```python
from build123d import *

# Parameters (mm, degrees)
SKETCH006_W   = 11.8
SKETCH006_H   = 11.8
PAD006_DEPTH  = 30
SKETCH001_R   = 40
SKETCH001_R_2 = 2.1
PAD001_DEPTH  = 5
PAD004_DEPTH  = 10.5
SKETCH005_R   = 2.1
PAD005_DEPTH  = 20
SKETCH_W      = 11.8
SKETCH_H      = 11.8
PAD_DEPTH     = 15


with BuildPart() as pad006:
    # Sketch006 → Pad006 (new body)
    with BuildSketch(Plane.XY):
        Rectangle(SKETCH006_W, SKETCH006_H)
    extrude(amount=PAD006_DEPTH)


with BuildPart() as pad001:
    # Sketch001 → Pad001 (new body)
    with BuildSketch(Plane.XY):
        Circle(SKETCH001_R)
        with Locations((0, 35)):
            Circle(SKETCH001_R_2, mode=Mode.SUBTRACT)
        with Locations((-35, 0)):
            Circle(SKETCH001_R_2, mode=Mode.SUBTRACT)
        with Locations((35, 0)):
            Circle(SKETCH001_R_2, mode=Mode.SUBTRACT)
        with Locations((0, -35)):
            Circle(SKETCH001_R_2, mode=Mode.SUBTRACT)
    extrude(amount=PAD001_DEPTH)


with BuildPart() as vis:
    # Cone → Cone (revolve)
    with BuildSketch(Plane(origin=(0, 0, 5), x_dir=(1, 0, 0), z_dir=(0, -1, 0))):
        Polygon((0, 0), (30, 0), (11.9, 9), (0, 9), align=None)
    revolve(axis=Axis((0, 0, 5), (0, 0, 1)))

    # Fusion001: union Pad001
    add(pad001.part)

    # Cut001: cut Pad006
    add(pad006.part, mode=Mode.SUBTRACT)


with BuildPart() as pad004:
    # Sketch004 → Pad004 (new body)
    with BuildSketch(Plane.XZ):
        Polygon((4.25, 24), (2.125, 27.680608), (-2.125, 27.680608), (-4.25, 24), (-2.125, 20.319392), (2.125, 20.319392), align=None)
    extrude(amount=PAD004_DEPTH)


with BuildPart() as screw_hole:
    # Sketch005 → Pad005 (new body)
    with BuildSketch(Plane.XZ):
        with Locations((0, 24)):
            Circle(SKETCH005_R)
    extrude(amount=PAD005_DEPTH)

    # Fusion: union Pad004
    add(pad004.part)


with BuildPart() as mobile:
    # Sketch → Pad (new body)
    with BuildSketch(Plane.XY.offset(15)):
        with BuildLine():
            ThreePointArc((7.5, -9.239048), (0, 11.9), (-7.5, -9.239048))
            Line((-7.5, -9.239048), (-7.5, -13.239048))
            Line((-7.5, -13.239048), (7.5, -13.239048))
            Line((7.5, -13.239048), (7.5, -9.239048))
        make_face()
        Rectangle(SKETCH_W, SKETCH_H, mode=Mode.SUBTRACT)
    extrude(amount=PAD_DEPTH)

    # Cut: cut screw_hole
    add(screw_hole.part, mode=Mode.SUBTRACT)


with BuildPart() as mobile_1:
    # Cut placement: moved
    add(mobile.part.moved(Location((0, 0, -4))))

    # Fusion002: union vis
    add(vis.part)


solid = mobile_1.part
```
The listing builds one solid part. Answer for the finished solid, in the listing's coordinates (mm). A direction names the side the tool comes from. Give positions to 0.01 mm unless a question says otherwise; leave off trailing zeros. Loops run counter-clockwise (first coordinate to the right, second up) from the corner with the lowest first, then second, coordinate; pieces in that order, holes last. Notation, with made-up numbers: (-36.5, 2) - (-6.5, 2) arc R24 cw to (-6.5, 17) - close; hole circle Ø4 at (64.5, 61). An arc over 180 degrees is marked (long way). Answer as CSV lines item,"result". Start each with the question number.
Item 1: A cutting plane is placed at D-D on y = -35. Determine the outline of the cut face in (x, z), then the cut area to 3 significant figures.
Item 2: A cutting plane is placed at C-C on x = 0. Count the separate pieces of the cut face and the enclosed holes in it, then the cut area to 3 significant figures.
Item 3: A cutting plane is placed at A-A on z = 24.75. Determine the outline of the cut face in (x, y), then the cut area to 3 significant figures.
Item 4: For faces 1 (the face through (0, 5.9, 13)), 2 (the face through (3.202, -8.168, 21.815)), 3 (the face through (0.41, 11.893, 19.916)), 4 (the face through (1.13, -11.85, 21.77)), determine the directions among +Z, -Z, +X, -X, +Y, -Y from which every point of the face is accessible in a straight line to the end or side of a thin tool.
Item 5: A cutting plane is placed at B-B on y = 0. Determine the outline of the cut face in (x, z), then the cut area to 3 significant figures.
Item 6: Each of these flat-tipped pins is pushed along its axis until it touches: pin 1 (1 mm diameter, centred on x = -1, y = 14.5, fed in from +Z); pin 2 (3.5 mm diameter, centred on x = 2, z = 19.5, fed in from +Y); pin 3 (13 mm diameter, centred on x = 2.5, z = 7, fed in from -Y); pin 4 (3.5 mm diameter, centred on x = 0, y = -35, fed in from -Z). Where does it stop, or does it pass through?
Item 7: The mould has two halves that part along Z. Classify faces 5 (the face through (9, -29, 5)), 6 (the face through (-7.5, -11, 19)), 7 (the face through (0, -8, 16.319)): +Z half, -Z half, draft (parallel to the pull), parting line (faces both ways), or undercut.
Item 8: Find the intervals of material crossed by line 1 (Y direction, x = 0, z = 2.8); line 2 (Z direction, x = 0, y = -11); line 3 (X direction, y = -0.5, z = 24.75), in increasing order. Write a range as from..to.
Found:
1,outline,"(-19.36, 0) - (-2.1, 0) - (-2.1, 5) - (-19.36, 5) - close; (2.1, 0) - (19.36, 0) - (19.36, 5) - (2.1, 5) - close"
1,area,"173 mm^2"
2,separate pieces,"5"
2,enclosed holes,"0"
2,area,"685 mm^2"
3,outline,"(-7.5, -13.24) - (7.5, -13.24) - (7.5, -9.24) arc R11.9 ccw (long way) to (-7.5, -9.24) - close; hole (-5.9, -5.9) - (5.9, -5.9) - (5.9, 5.9) - (-5.9, 5.9) - close"
3,area,"338 mm^2"
4,face 1,"+Z, -Z"
4,face 2,"none"
4,face 3,"+Z"
4,face 4,"-Y"
5,outline,"(-40, 0) - (-37.1, 0) - (-37.1, 5) - (-40, 5) - close; (-32.9, 0) - (-5.9, 0) - (-5.9, 26) - (-11.9, 26) - (-11.9, 14) - (-30, 5) - (-32.9, 5) - close; (5.9, 0) - (32.9, 0) - (32.9, 5) - (30, 5) - (11.9, 14) - (11.9, 26) - (5.9, 26) - close; (37.1, 0) - (40, 0) - (40, 5) - (37.1, 5) - close"
5,area,"714 mm^2"
6,pin 1,"stops at z = 12.94"
6,pin 2,"stops at y = 11.9"
6,pin 3,"stops at y = -40"
6,pin 4,"passes through"
7,face 5,"+Z half"
7,face 6,"draft"
7,face 7,"undercut"
8,line 1,"y = -40..-37.1, -32.9..-5.9, 5.9..32.9, 37.1..40"
8,line 2,"z = 0..17.9, 22.1..26"
8,line 3,"x = -11.89..-5.9, 5.9..11.89"
